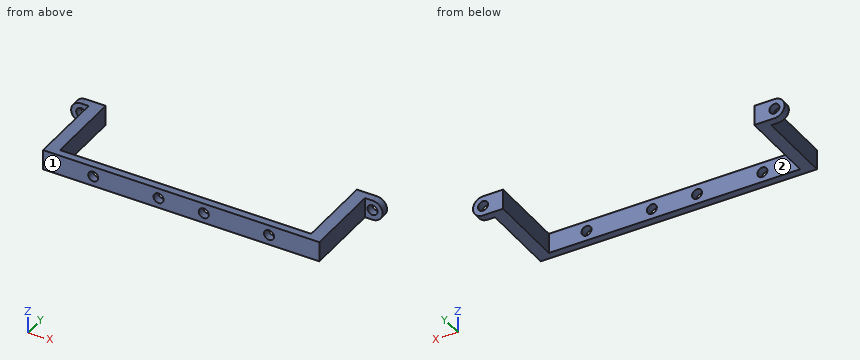
```python
from build123d import *

# Parameters (mm, degrees)
SKETCH1_W           = 110
SKETCH1_H           = 8
SKETCH1_R           = 2
BOSS_EXTRUDE1_DEPTH = 3
SKETCH2_W           = 5
SKETCH2_H           = 8
BOSS_EXTRUDE2_DEPTH = 28
SKETCH3_R           = 2
BOSS_EXTRUDE3_DEPTH = 3


with BuildPart() as part:
    # Sketch1 → Boss-Extrude1 (new body)
    with BuildSketch(Plane(origin=(0, 0, 0), x_dir=(1, 0, 0), z_dir=(0, 1, 0))):
        Rectangle(SKETCH1_W, SKETCH1_H)
        with Locations(Location((-35, 0, 0), (0, 0, 270))):
            Circle(SKETCH1_R, mode=Mode.SUBTRACT)
        with Locations(Location((35, 0, 0), (0, 0, 270))):
            Circle(SKETCH1_R, mode=Mode.SUBTRACT)
        with Locations(Location((-9, 0, 0), (0, 0, 270))):
            Circle(SKETCH1_R, mode=Mode.SUBTRACT)
        with Locations(Location((9, 0, 0), (0, 0, 270))):
            Circle(SKETCH1_R, mode=Mode.SUBTRACT)
    extrude(amount=BOSS_EXTRUDE1_DEPTH)

    # Sketch2 → Boss-Extrude2 (add)
    with BuildSketch(Plane(origin=(0, 3, 0), x_dir=(1, 0, 0), z_dir=(0, 1, 0))):
        with Locations((-52.5, 0)):
            Rectangle(SKETCH2_W, SKETCH2_H)
        with Locations((52.5, 0)):
            Rectangle(SKETCH2_W, SKETCH2_H)
    extrude(amount=BOSS_EXTRUDE2_DEPTH)

    # Sketch3 → Boss-Extrude3 (add)
    # profile 1 of 2: a face of its own
    with BuildSketch(Plane(origin=(0, 31, 0), x_dir=(1, 0, 0), z_dir=(0, 1, 0))):
        with BuildLine():
            Line((-50, 4), (-58, 4))
            ThreePointArc((-58, 4), (-62, 0), (-58, -4))
            Line((-58, -4), (-50, -4))
            Line((-50, -4), (-50, 4))
        make_face()
        with Locations(Location((-58, 0, 0), (0, 0, 270))):
            Circle(SKETCH3_R, mode=Mode.SUBTRACT)
    # profile 2 of 2: a face of its own
    with BuildSketch(Plane(origin=(0, 31, 0), x_dir=(1, 0, 0), z_dir=(0, 1, 0))):
        with BuildLine():
            Line((50, 4), (58, 4))
            ThreePointArc((58, 4), (62, 0), (58, -4))
            Line((58, -4), (50, -4))
            Line((50, -4), (50, 4))
        make_face()
        with Locations(Location((58, 0, 0), (0, 0, 90))):
            Circle(SKETCH3_R, mode=Mode.SUBTRACT)
    extrude(amount=BOSS_EXTRUDE3_DEPTH)


solid = part.part
```
Can you work these out from the model? Positions are in its coordinate system, mm. Face numbers are marked on the shaded views. Give positions to 0.01 mm unless a question says otherwise; leave off trailing zeros. Write each loop counter-clockwise with the first axis right and the second up, starting at its lowest first coordinate (ties: lowest second). Pieces come first, ordered by that corner, then holes. Notation, with made-up numbers: (-36.75, -16.5) - (13.25, -16.5) arc R35 cw to (13.25, 22.5) - close; hole circle Ø7 at (-3.75, 66.25). An arc over 180 degrees is marked (long way). Write item = value, one per line. Start each with the question number.
1. Thinking about a two-plate mould opening in X: for the marked faces 1 and 2, which applies, released by +X, released by -X, zero draft, split by the parting line, or undercut?
2. Imagine slicing it at D-D (x = 38.5). Please give me the cut outline in (y, z), and give its area (3 significant figures).
3. Imagine slicing it at C-C (z = 0). Count the separate pieces of the cut face and the enclosed holes in it, and give its area (3 significant figures).
4. Imagine slicing it at A-A (y = 27.5). Please give me the cut outline in (x, z), and give its area (3 significant figures).
5. Please list where these lines run through material, in increasing order: line 1 (X direction, y = 31.6, z = 0); line 2 (X direction, y = 0.65, z = 0); line 3 (X direction, y = 26.5, z = 0).
6. For pin 1 (1 mm diameter, centred on x = -33.5, z = -2.5, fed in from -Y); pin 2 (2 mm diameter, centred on y = 7, z = 0.5, fed in from -X); pin 3 (4.5 mm diameter, centred on x = -9, z = 0, fed in from +Y); pin 4 (2.5 mm diameter, centred on x = -35, z = 0, fed in from -Y), each with a flat end and sliding along its axis, tell me the tip position at first contact or that it passes through.
7. Imagine slicing it at B-B (x = -35). Please give me the cut outline in (y, z), and give its area (3 significant figures).
Worked answers:
q1.face_1 = zero draft
q1.face_2 = undercut
q2.outline = (0, -4) - (3, -4) - (3, 4) - (0, 4) - close
q2.area = 24.0 mm2
q3.separate_pieces = 7
q3.enclosed_holes = 0
q3.area = 610 mm2
q4.outline = (-55, -4) - (-50, -4) - (-50, 4) - (-55, 4) - close; (50, -4) - (55, -4) - (55, 4) - (50, 4) - close
q4.area = 80.0 mm2
q5.line_1 = -62 to -60, -56 to -50, 50 to 56, 60 to 62
q5.line_2 = -55 to -37, -33 to -11, -7 to 7, 11 to 33, 37 to 55
q5.line_3 = -55 to -50, 50 to 55
q6.pin_1 = 0
q6.pin_2 = -55
q6.pin_3 = 3
q6.pin_4 = through
q7.outline = (0, -4) - (3, -4) - (3, -2) - (0, -2) - close; (0, 2) - (3, 2) - (3, 4) - (0, 4) - close
q7.area = 12.0 mm2
